from build123d import *

# Parameters (mm, degrees)
BOSS_EXTRUDE2_DEPTH      = 150
SHELL1_T                 = -5
BOSS_EXTRUDE4_DEPTH      = 5
BOSS_EXTRUDE4_DEPTH_BACK = 5
SKETCH2_R                = 2.5
BOSS_EXTRUDE5_DEPTH      = 5
BOSS_EXTRUDE5_DEPTH_BACK = 5
SKETCH3_R                = 2.5
SKETCH4_R                = 2.5
BOSS_EXTRUDE7_DEPTH      = 2.5
BOSS_EXTRUDE8_DEPTH      = 5.5
SKETCH7_R                = 0.75
CUT_EXTRUDE1_DEPTH       = 5.5


with BuildPart() as part:
    # Sketch1 → Boss-Extrude2 (new body)
    with BuildSketch(Plane.XY):
        Polygon((0, 150), (0, 135), (35, 135), (121.711027725, 26.105238444), (320, 0), (320, 150), align=None)
    extrude(amount=BOSS_EXTRUDE2_DEPTH)

    # Shell1
    shell1_openings = [part.faces().sort_by_distance(p)[0] for p in [
        (160, 150, 75),
        (320, 75, 75),
    ]]
    offset(amount=SHELL1_T, openings=shell1_openings, kind=Kind.INTERSECTION)

    # Sketch2 → Boss-Extrude4 (add, two sides: drawn at the far end of the back side and taken through both)
    with BuildSketch(Plane.XY.offset(150).offset(-BOSS_EXTRUDE4_DEPTH_BACK)):
        with Locations((320, 150)):
            Circle(SKETCH2_R)
    extrude(amount=BOSS_EXTRUDE4_DEPTH + BOSS_EXTRUDE4_DEPTH_BACK)

    # Sketch3 → Boss-Extrude5 (add, two sides: drawn at the far end of the back side and taken through both)
    with BuildSketch(Plane(origin=(0, 0, 0), x_dir=(-1, 0, 0), z_dir=(0, 0, -1)).offset(-BOSS_EXTRUDE5_DEPTH_BACK)):
        with Locations(Location((-320, 150, 0), (0, 0, 180))):
            Circle(SKETCH3_R)
    extrude(amount=BOSS_EXTRUDE5_DEPTH + BOSS_EXTRUDE5_DEPTH_BACK)

    # Sketch4 → Boss-Extrude7 (add)
    with BuildSketch(Plane.XY.offset(150)):
        with Locations(Location((320, 0, 0), (0, 0, 172.5))):
            Circle(SKETCH4_R)
    boss_extrude7 = extrude(amount=BOSS_EXTRUDE7_DEPTH)

    # Mirror1: Boss-Extrude7 across plane
    add(boss_extrude7.mirror(Plane.XY.offset(75)))

    # Sketch6 → Boss-Extrude8 (add)
    with BuildSketch(Plane.XZ.offset(-135)):
        Polygon((17.733333333, 74), (17.266666667, 76), (16.25, 76), (16.25, 74), align=None)
        Polygon((18.75, 76), (17.266666667, 76), (17.733333333, 74), (18.75, 74), align=None)
    extrude(amount=BOSS_EXTRUDE8_DEPTH)

    # Sketch7 → Cut-Extrude1 (cut)
    with BuildSketch(Plane.XY.offset(76)):
        with Locations((17.5, 131)):
            Circle(SKETCH7_R)
        with BuildLine():
            Line((16.25, 135), (16.501917688, 130.938099278))
            ThreePointArc((16.501917688, 130.938099278), (17.5, 130), (18.498082312, 130.938099278))
            Line((18.498082312, 130.938099278), (18.75, 135))
            Line((18.75, 135), (18.75, 129.5))
            Line((18.75, 129.5), (16.25, 129.5))
            Line((16.25, 129.5), (16.25, 135))
        make_face()
    extrude(amount=-CUT_EXTRUDE1_DEPTH, mode=Mode.SUBTRACT)


solid = part.part
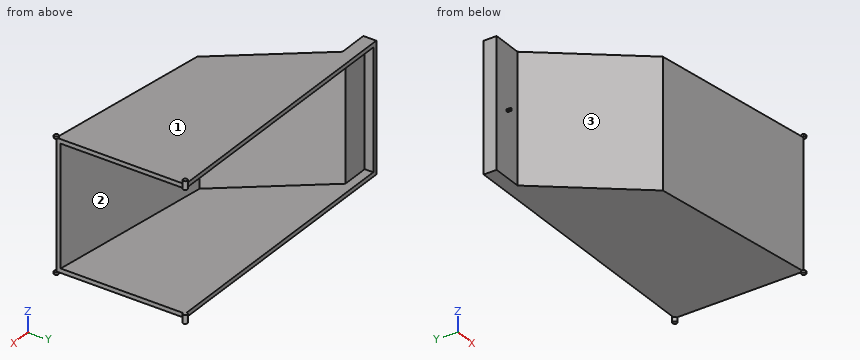
Design review of the part built by this model. Coordinates are the model's own, in mm. Face numbers are marked on the shaded views. Give positions to 0.01 mm unless a question says otherwise; leave off trailing zeros. Order: outer loops, then holes, each group sorted by start corner. A loop starts at its lowest first (then second) coordinate and runs counter-clockwise, first axis right, second up. Notation, with made-up numbers: (-22.5, 84) - (34.5, 84) arc R30 ccw to (34.5, 120) - close; hole circle Ø8 at (3.5, 17.25). An arc over 180 degrees is marked (long way). Use CSV: the item, a comma, the result in double quotes. Start each with the question number.
Q1. Take a section at B-B (z = 46.5). State the section outline as (x, y) points.
Q2. Take a section at A-A (x = 229). State the section outline as (y, z) points, and give its area (3 significant figures).
Q3. For P1, Ø6, axis at x = 159, z = 15.5, coming from the +Y side; P2, Ø3, axis at x = 162, y = 68.5, coming from the +Z side; P3, Ø3, axis at y = 48, z = 28, coming from the +X side, all flat-tipped, find the tip position at first contact; note any pin that passes through.
Q4. For line 1 (Z direction, x = 147.5, y = 99); line 2 (X direction, y = 131, z = 74.4); line 3 (Y direction, x = 17.5, z = 74.6), list the stretches that pass through material, from the lowest coordinate up.
Q5. Take a section at C-C (y = 55). State the section outline as (x, z) points, and give its area (3 significant figures).
Q6. Draft analysis for pull direction Z (two halves, no side actions). For the marked faces 1, 2 and 3, state which applies: pulls with the +Z half, pulls with the -Z half, needs draft (parallel to the pull), parting line crosses it, or undercut.
Calculated:
1,outline,"(0, 135) - (35, 135) - (121.71, 26.11) - (320, 0) - (320, 5.04) - (124.37, 30.8) - (37.41, 140) - (5, 140) - (5, 150) - (0, 150) - close"
2,outline,"(11.98, 0) - (150, 0) - (150, 5) - (17.02, 5) - (17.02, 145) - (150, 145) - (150, 150) - (11.98, 150) - close"
2,area,"2,090 mm²"
3,P1,"stops at y = 26.63"
3,P2,"stops at z = 150"
3,P3,"stops at x = 111.86"
4,line 1,"z = 0 to 5, 145 to 150"
4,line 2,"x = 16.5 to 16.75, 18.25 to 18.5, 38.19 to 44.58"
4,line 3,"y = 130 to 130.25, 131.75 to 140"
5,outline,"(98.7, 0) - (320, 0) - (320, 5) - (105.09, 5) - (105.09, 145) - (320, 145) - (320, 150) - (98.7, 150) - close"
5,area,"3,110 mm²"
6,face 1,"pulls with the +Z half"
6,face 2,"undercut"
6,face 3,"needs draft"
